```python
from build123d import *

# Parameters (mm, degrees)
SKETCH_1_R          = 2.4
SKETCH_1_R_2        = 6.5
EXTRUDE_1_DEPTH     = 40
FILLET_1_R          = 10
SKETCH_2_R          = 2.4
CUT_EXTRUDE_1_DEPTH = 66.0828238
SKETCH_4_R          = 41.2
CUT_EXTRUDE_2_DEPTH = 5.5
CUT_EXTRUDE_3_DEPTH = 64.25167155


with BuildPart() as part:
    # 草图1 → 凸台-拉伸1 (new body)
    with BuildSketch(Plane.XY):
        Polygon((-29.269334238, -5), (44.269334238, -5), (36.813954208, 21), (-21.813954208, 21), align=None)
        with Locations((15, 17)):
            Circle(SKETCH_1_R, mode=Mode.SUBTRACT)
        with Locations((15, 0)):
            Circle(SKETCH_1_R, mode=Mode.SUBTRACT)
        Circle(SKETCH_1_R, mode=Mode.SUBTRACT)
        with Locations((0, 17)):
            Circle(SKETCH_1_R, mode=Mode.SUBTRACT)
        with Locations((7.5, 8)):
            Circle(SKETCH_1_R_2, mode=Mode.SUBTRACT)
    extrude(amount=EXTRUDE_1_DEPTH)

    # 圆角1
    fillet_1_edges = [part.edges().sort_by_distance(p)[0] for p in [
        (-21.813954208, 21, 20),
        (36.813954208, 21, 20),
    ]]
    fillet(fillet_1_edges, radius=FILLET_1_R)

    # 草图2 → 切除-拉伸1 (cut, through all)
    with BuildSketch(Plane(origin=(0, 21, 0), x_dir=(1, 0, 0), z_dir=(0, 1, 0))):
        with Locations(Location((-5, -5, 0), (0, 0, 180))):
            Circle(SKETCH_2_R)
        with Locations(Location((20, -5, 0), (0, 0, 180))):
            Circle(SKETCH_2_R)
        with Locations(Location((-5, -35, 0), (0, 0, 180))):
            Circle(SKETCH_2_R)
        with Locations(Location((20, -35, 0), (0, 0, 180))):
            Circle(SKETCH_2_R)
    extrude(amount=-CUT_EXTRUDE_1_DEPTH, mode=Mode.SUBTRACT)

    # 草图4 → 切除-拉伸2 (cut)
    with BuildSketch(Plane.XY.offset(40)):
        with Locations((-46.5, 45)):
            Circle(SKETCH_4_R)
        with Locations((61.5, 45)):
            Circle(SKETCH_4_R)
    extrude(amount=-CUT_EXTRUDE_2_DEPTH, mode=Mode.SUBTRACT)

    # 草图5 → 切除-拉伸3 (cut, through all)
    with BuildSketch(Plane(origin=(0, 0, 0), x_dir=(-1, 0, 0), z_dir=(0, 0, -1))):
        Polygon((-42.269334238, -5), (-44.269334238, -5), (-43.695843466, -3), align=None)
        Polygon((28.695843466, -3), (27.269334238, -5), (29.269334238, -5), align=None)
    extrude(amount=-CUT_EXTRUDE_3_DEPTH, mode=Mode.SUBTRACT)


solid = part.part
```
Input: part model. Units: mm. Frame: model coordinates. A direction names the side the tool comes from. Coordinates: 2 decimals unless noted, no trailing zeros. Order: outer loops, then holes, each group sorted by start corner. A loop starts at its lowest first (then second) coordinate and runs counter-clockwise, first axis right, second up. Notation, with made-up numbers: (13, 34.25) - (68, 34.25) arc R20 ccw to (68, 46.25) - close; hole circle Ø9 at (27, 61.25). An arc over 180 degrees is marked (long way). Put each result on its own line as item: value.
1. Reachability of faces 1 (the face through (35, 16, 34.5)), 2 (the face through (7, -5, 20)), 3 (the face through (-18.54, 14.74, 37.29)) from +Z, -Z, +X, -X, +Y, -Y: full face, straight path, thin tool, end or side. Return the list, or none.
Report:
face 1: +Z, +X, +Y
face 2: +Z, -Z, +X, -X, -Y
face 3: +Z, -X, +Y
2. Cut plane C-C on y = 17. Return the cut outline in (x, z).
Report:
outline: (-22.28, 0) - (-2.4, 0) - (-2.4, 40) - (-16.28, 40) - (-16.28, 34.5) - (-22.28, 34.5) - close; (2.4, 0) - (12.6, 0) - (12.6, 40) - (2.4, 40) - close; (17.4, 0) - (37.28, 0) - (37.28, 34.5) - (31.28, 34.5) - (31.28, 40) - (17.4, 40) - close; hole circle Ø4.8 at (-5, 5); hole circle Ø4.8 at (-5, 35); hole circle Ø4.8 at (20, 5); hole circle Ø4.8 at (20, 35)
3. Contact query for flat-ended pins moving along their axis: pin 1 Ø1 at (y, z) = (13.5, 14) entering from +X; pin 2 Ø1.5 at (y, z) = (5.5, 28) entering from +X; pin 3 Ø6 at (y, z) = (11.5, 17) entering from +X. Output: stop coordinate, or through.
Report:
pin 1: stops at x = 39.11
pin 2: stops at x = 41.47
pin 3: stops at x = 40.4
4. Cut plane A-A on x = 20. Return the cut outline in (y, z).
Report:
outline: (-5, 0) - (21, 0) - (21, 2.6) - (-5, 2.6) - close; (-5, 7.4) - (21, 7.4) - (21, 32.6) - (-5, 32.6) - close; (-5, 37.4) - (21, 37.4) - (21, 40) - (-5, 40) - close
5. Line query: line 1 along Y through (x, z) = (0, 37.5); line 2 along Z through (x, y) = (20, 12.5); line 3 along X through (y, z) = (-0.75, 14). Output: solid intervals per line, ascending.
Report:
line 1: y = -5 to -2.4, 2.4 to 14.6, 19.4 to 21
line 2: z = 0 to 2.6, 7.4 to 32.6, 37.4 to 40
line 3: x = -28.05 to -2.28, 2.28 to 12.72, 17.28 to 43.05
6. Cut plane D-D on y = 8. Return the cut outline in (x, z), then the cut area to 3 significant figures.
Report:
outline: (-25.54, 0) - (1, 0) - (1, 40) - (-25.54, 40) - close; (14, 0) - (40.54, 0) - (40.54, 40) - (14, 40) - close; hole circle Ø4.8 at (-5, 5); hole circle Ø4.8 at (-5, 35); hole circle Ø4.8 at (20, 5); hole circle Ø4.8 at (20, 35)
area: 2,050 mm2
7. Cut plane B-B on z = 5. Return the cut outline in (x, y), then the cut area to 3 significant figures.
Report:
outline: (-28.7, -3) - (-27.27, -5) - (-7.4, -5) - (-7.4, 21) - (-14.28, 21) arc R10 ccw to (-23.89, 13.76) - close; (-2.6, -5) - (17.6, -5) - (17.6, 21) - (-2.6, 21) - close; (22.4, -5) - (42.27, -5) - (43.7, -3) - (38.89, 13.76) arc R10 ccw to (29.28, 21) - (22.4, 21) - close; hole circle Ø4.8 at (0, 0); hole circle Ø4.8 at (0, 17); hole circle Ø13 at (7.5, 8); hole circle Ø4.8 at (15, 0); hole circle Ø4.8 at (15, 17)
area: 1,240 mm2
8. Draft query along X for faces 4 (the face through (-27.99, -3.99, 19.72)), 5 (the face through (35.37, 18.93, 17.49)), 6 (the face through (12.602, 0.106, 19.72)). Return one class per face: pulls with the +X half, pulls with the -X half, needs draft (parallel to the pull), parting line crosses it, or undercut.
Report:
face 4: pulls with the -X half
face 5: pulls with the +X half
face 6: undercut
